Source: CAD feature listing. Evaluate the final solid. Frame: model axes, mm. Round coordinates to 2 decimals unless told otherwise and drop trailing zeros. Write each loop counter-clockwise with the first axis right and the second up, starting at its lowest first coordinate (ties: lowest second). Pieces come first, ordered by that corner, then holes. Notation, with made-up numbers: M 44,-3.5 L 67,-3.5 A15 cw 67,0.5 Z; hole C 49,-11.5 d1. An arc over 180 degrees is marked long. Answer in a Markdown table with one row per item. Add a question column.
Item 1: Mould query, pull axis X, two halves, no side actions, for faces 1 (the face through (7.6, 0.8, -7.2)), 2 (the face through (8.89, 1, 0)), 3 (the face through (0, 1, -9.525)), 4 (the face through (-8.289, 0.789, 8.955)). Classes: released by +X, released by -X, zero draft, split by the parting line, or undercut.
Item 2: Material intervals for probe 1 along X at (y, z) = (1.5, -7); probe 2 along X at (y, z) = (1.3, -8.5); probe 3 along Z at (x, y) = (-7, 0.3), sorted ascending.
Item 3: Contact query for flat-ended pins moving along their axis: pin 1 (1.5 mm diameter, centred on x = -6.35, z = -6.985, fed in from +Y); pin 2 (6 mm diameter, centred on x = 2, z = 5, fed in from -Y). Output: stop coordinate, or through.
Item 4: Cut plane C-C on z = -6.25. Return loops of the section in (x, y), and give its area (3 significant figures).
Item 5: Cut plane A-A on x = -6.35. Return loops of the section in (y, z) (3 decimals), and give its area (3 significant figures).
Item 6: Cut plane B-B on y = 0.9. Return loops of the section in (x, z) (3 decimals), and give its area (3 significant figures).
from build123d import *

# Parameters (mm, degrees)
BOSS_EXTRUDE1_DEPTH = 1.6
SKETCH2_R           = 1.27
CUT_EXTRUDE1_DEPTH  = 1.6


with BuildPart() as part:
    # Sketch1 → Boss-Extrude1 (new body)
    with BuildSketch(Plane(origin=(0, 0, 0), x_dir=(1, 0, 0), z_dir=(0, 1, 0))):
        with BuildLine():
            Line((-6.89, 9.525), (6.89, 9.525))
            ThreePointArc((6.89, 9.525), (8.304213562, 8.939213562), (8.89, 7.525))
            Line((8.89, 7.525), (8.89, -7.525))
            ThreePointArc((8.89, -7.525), (8.304213562, -8.939213562), (6.89, -9.525))
            Line((6.89, -9.525), (-6.89, -9.525))
            ThreePointArc((-6.89, -9.525), (-8.304213562, -8.939213562), (-8.89, -7.525))
            Line((-8.89, -7.525), (-8.89, 7.525))
            ThreePointArc((-8.89, 7.525), (-8.304213562, 8.939213562), (-6.89, 9.525))
        make_face()
    extrude(amount=BOSS_EXTRUDE1_DEPTH)

    # Sketch2 → Cut-Extrude1 (cut)
    with BuildSketch(Plane(origin=(0, 1.6, 0), x_dir=(1, 0, 0), z_dir=(0, 1, 0))):
        with Locations(Location((-6.35, 6.985, 0), (0, 0, 270))):
            Circle(SKETCH2_R)
        with Locations(Location((6.35, 6.985, 0), (0, 0, 270))):
            Circle(SKETCH2_R)
    extrude(amount=-CUT_EXTRUDE1_DEPTH, mode=Mode.SUBTRACT)


solid = part.part
Results below:
| question | item | result |
|---|---|---|
| 1 | face 1 | undercut |
| 1 | face 2 | released by +X |
| 1 | face 3 | zero draft |
| 1 | face 4 | released by -X |
| 2 | probe 1 | -8.89 to -7.62, -5.08 to 5.08, 7.62 to 8.89 |
| 2 | probe 2 | -8.64 to 8.64 |
| 2 | probe 3 | -9.52 to -8.08, -5.89 to 9.52 |
| 3 | pin 1 | through |
| 3 | pin 2 | y = 0 |
| 4 | outline | M -8.89,0 L -7.39,0 L -7.39,1.6 L -8.89,1.6 Z; M -5.31,0 L 5.31,0 L 5.31,1.6 L -5.31,1.6 Z; M 7.39,0 L 8.89,0 L 8.89,1.6 L 7.39,1.6 Z |
| 4 | area | 21.8 mm2 |
| 5 | outline | M 0,-9.525 L 1.6,-9.525 L 1.6,-8.255 L 0,-8.255 Z; M 0,-5.715 L 1.6,-5.715 L 1.6,9.525 L 0,9.525 Z |
| 5 | area | 26.4 mm2 |
| 6 | outline | M -8.89,-7.525 A2 ccw -6.89,-9.525 L 6.89,-9.525 A2 ccw 8.89,-7.525 L 8.89,7.525 A2 ccw 6.89,9.525 L -6.89,9.525 A2 ccw -8.89,7.525 Z; hole C -6.35,-6.985 d2.54; hole C 6.35,-6.985 d2.54 |
| 6 | area | 325 mm2 |
